Source: CAD feature listing. Evaluate the final solid. Frame: model axes, mm. Face numbers are marked on the shaded views. A direction names the side the tool comes from. Coordinates: 2 decimals unless noted, no trailing zeros. Write each loop counter-clockwise with the first axis right and the second up, starting at its lowest first coordinate (ties: lowest second). Pieces come first, ordered by that corner, then holes. Notation, with made-up numbers: (21, 87) -> (55, 87) arc R28 ccw to (55, 122) -> close; hole circle Ø11 at (-8.5, 16.5). An arc over 180 degrees is marked (long way). Write item = value, one per line.
from build123d import *

# Parameters (mm, degrees)
BOSS_EXTRUDE1_DEPTH = 17
SKETCH2_R           = 2.2
CUT_EXTRUDE1_DEPTH  = 17


with BuildPart() as part:
    # Sketch1 → Boss-Extrude1 (new body)
    with BuildSketch(Plane(origin=(0, 0, 0), x_dir=(1, 0, 0), z_dir=(0, 1, 0))):
        Polygon((0, 0), (0, 11), (18, 11), (18, 0), (15, 0), (15, 8), (3, 8), (3, 0), align=None)
    extrude(amount=BOSS_EXTRUDE1_DEPTH)

    # Sketch2 → Cut-Extrude1 (cut)
    with BuildSketch(Plane(origin=(0, 0, -11), x_dir=(-1, 0, 0), z_dir=(0, 0, -1))):
        with Locations((-9, 8.5)):
            Circle(SKETCH2_R)
    extrude(amount=-CUT_EXTRUDE1_DEPTH, mode=Mode.SUBTRACT)


solid = part.part
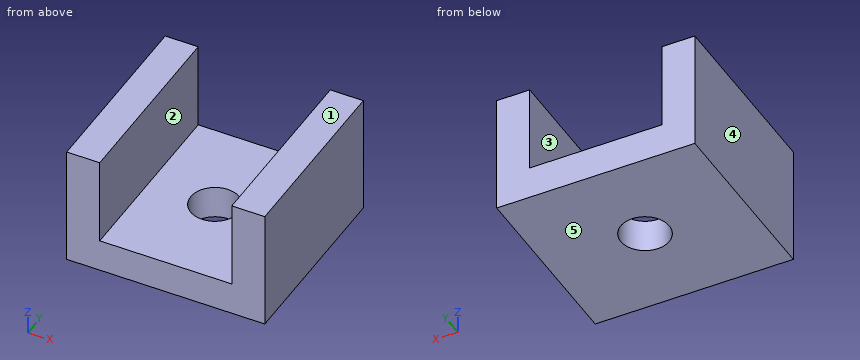
1) Reachability of the marked faces 1 and 2 from +Z, -Z, +X, -X, +Y, -Y: full face, straight path, thin tool, end or side. Return the list, or none.
Answer block:
face_1 = +Z, +X, -X, +Y, -Y
face_2 = +Z, +Y, -Y
2) First-contact query: pin 1 Ø5.5 at (x, y) = (9, 8.5) entering from +Z; pin 2 Ø1 at (x, z) = (4, -5.5) entering from -Y. Flat tips, straight axial feed; report the tip coordinate or a pass-through.
Answer block:
pin_1 = -8
pin_2 = through
3) Cut plane A-A, the plane x = 9. Output: boundary loops of the cut face in (y, z).
Answer block:
outline = (0, -11) -> (6.3, -11) -> (6.3, -8) -> (0, -8) -> close; (10.7, -11) -> (17, -11) -> (17, -8) -> (10.7, -8) -> close
4) Pull-direction query (X, two-part tool) for the marked faces 3, 4 and 5; classes: +X half, -X half, draft (parallel to the pull), parting line (faces both ways), or undercut.
Answer block:
face_3 = undercut
face_4 = -X half
face_5 = draft
5) Cut plane D-D, the plane z = -9.25. Output: boundary loops of the cut face in (x, y).
Answer block:
outline = (0, 0) -> (18, 0) -> (18, 17) -> (0, 17) -> close; hole circle Ø4.4 at (9, 8.5)
6) Material intervals for probe 1 along X at (y, z) = (1.25, -1.5); probe 2 along Y at (x, z) = (9, -9.4); probe 3 along Z at (x, y) = (6.5, 16), sorted ascending. Write a range as [from, to].
Answer block:
probe_1 = [0, 3], [15, 18]
probe_2 = [0, 6.3], [10.7, 17]
probe_3 = [-11, -8]
7) Cut plane C-C, the plane z = -1.5. Output: boundary loops of the cut face in (x, y), and give its area (3 significant figures).
Answer block:
outline = (0, 0) -> (3, 0) -> (3, 17) -> (0, 17) -> close; (15, 0) -> (18, 0) -> (18, 17) -> (15, 17) -> close
area = 102 mm2
8) Cut plane B-B, the plane y = 8.5. Output: boundary loops of the cut face in (x, z), and give its area (3 significant figures).
Answer block:
outline = (0, -11) -> (6.8, -11) -> (6.8, -8) -> (3, -8) -> (3, 0) -> (0, 0) -> close; (11.2, -11) -> (18, -11) -> (18, 0) -> (15, 0) -> (15, -8) -> (11.2, -8) -> close
area = 88.8 mm2
